Part model, mm, in its own coordinate system. A direction names the side the tool comes from. Give positions to 0.01 mm unless a question says otherwise; leave off trailing zeros. Order: outer loops, then holes, each group sorted by start corner. A loop starts at its lowest first (then second) coordinate and runs counter-clockwise, first axis right, second up. Notation, with made-up numbers: (70, -28) - (93, -28) arc R17 ccw to (93, -9) - close; hole circle Ø11 at (40, -1.75). An arc over 180 degrees is marked (long way). Use one line per item in the form item = value. Start each with the question number.
1. Pull direction Z, two halves, no side cores. Call faces 1 (the face through (4, -4.3, 11)), 2 (the face through (0.91, -1.11, -14.18)), 3 (the face through (4, 0, 34)), 4 (the face through (1.203, -0.599, 45.859)): +Z half, -Z half, draft (parallel to the pull), parting line (faces both ways), or undercut.
2. Drill centre lines: line 1 (Z direction, x = 4, y = 1.4); line 2 (Z direction, x = 7, y = -2.5); line 3 (Y direction, x = 5.25, z = -23.5). Where is each one in solid material? Low to high.
3. Tool access for faces 5 (the face through (4.195, -2.12, 14.502)), 6 (the face through (3.317, 2.696, 39.925)), 7 (the face through (4, -4.3, 41)), 8 (the face through (5, -4.3, -14)): list every direction of +Z, -Z, +X, -X, +Y, -Y with a clear straight run to the whole face (end or side of a thin tool).
4. Band-saw the part on B-B, the plane z = 4.75. List the corners of the cut face in (x, y).
5. Band-saw the part on A-A, the plane z = 13. List the corners of the cut face in (x, y), plus the area to 3 significant figures.
6. Pin check, flat tips, straight feed: P1, Ø4, axis at y = -5.5, z = 16, coming from the -X side; P2, Ø4, axis at x = 2.5, z = -21.5, coming from the -Y side. Stop position of each tip, or through.
from build123d import *

# Parameters (mm, degrees)
F0_R      = 1.5
F3_DEPTH  = 3
F0_R_2    = 3.15
F5_DEPTH  = 3
F6_DEPTH  = 4.3
F7_DEPTH  = 7.8
F8_DEPTH  = 0.8
F1_R      = 2.25
F9_DEPTH  = 88
F10_DEPTH = 0.8
F12_R     = 1
F13_DEPTH = 2.4


# Not quite as in the source:
# - an extrude ends at something that could not be found from the text; its depth is read off the source's solid


with BuildPart() as f3:
    # F0 (on Front) → F3 (new body)
    with BuildSketch(Plane.XZ):
        with BuildLine():
            Line((8.25, -28), (8.25, 0))
            Line((8.25, 0), (0, 0))
            ThreePointArc((0, 0), (0.9337479911, -14.3772966716), (3.7193040011, -28.5130394045))
            ThreePointArc((3.7193040011, -28.5130394045), (4.4329720676, -29.5852568891), (5.6523820051, -30))
            Line((5.6523820051, -30), (6.25, -30))
            ThreePointArc((6.25, -30), (7.6642135624, -29.4142135624), (8.25, -28))
        make_face()
        with Locations((4.125, -5)):
            Circle(F0_R, mode=Mode.SUBTRACT)
    extrude(amount=-F3_DEPTH)

    # F4: sweep along a path in F4_path
    with BuildLine(Plane(origin=(3.7193040011, 3, -28.5130394045), x_dir=(0, 0, 1), z_dir=(0, -1, 0))) as f4_path:
        ThreePointArc((28.5130394045, 3.7193040011), (14.1357427329, 2.78555601), (0, 0))
        ThreePointArc((0, 0), (-1.0722174846, -0.7136680665), (-1.4869605955, -1.933078004))
        Line((-1.4869605955, -1.933078004), (-1.4869605955, -2.5306959989))
        ThreePointArc((-1.4869605955, -2.5306959989), (-0.9011741579, -3.9449095613), (0.5130394045, -4.5306959989))
        Line((0.5130394045, -4.5306959989), (28.5130394045, -4.5306959989))
    # F2 (on Top) → F4 (sweep, cut)
    with BuildSketch(Plane.XY):
        with BuildLine():
            ThreePointArc((7.25, 3), (7.9571067812, 2.7071067812), (8.25, 2))
            Line((8.25, 2), (8.25, 3))
            Line((8.25, 3), (7.25, 3))
        make_face()
    sweep(path=f4_path.line, mode=Mode.SUBTRACT)

    # F0 (on Front) → F5 (join, through all)
    with BuildSketch(Plane.XZ):
        with BuildLine():
            Line((8.25, 0), (8.25, 15.324121816))
            ThreePointArc((8.25, 15.324121816), (4.1356957298, 14.5011227991), (0, 15.2088288402))
            Line((0, 15.2088288402), (0, 0))
            Line((0, 0), (8.25, 0))
        make_face()
        with BuildLine():
            Line((8.25, 15.324121816), (8.25, 23.4068600115))
            ThreePointArc((8.25, 23.4068600115), (4.2412321866, 21.0070929888), (0, 22.9669528523))
            Line((0, 22.9669528523), (0, 15.2088288402))
            ThreePointArc((0, 15.2088288402), (4.1356957298, 14.5011227991), (8.25, 15.324121816))
        make_face()
        with BuildLine():
            Line((8.25, 23.4068600115), (8.25, 26))
            Line((8.25, 26), (7.95, 26))
            ThreePointArc((7.95, 26), (3.975, 22.025), (0, 26))
            Line((0, 26), (0, 22.9669528523))
            ThreePointArc((0, 22.9669528523), (4.2412321866, 21.0070929888), (8.25, 23.4068600115))
        make_face()
        with BuildLine():
            ThreePointArc((7.95, 26), (3.975, 29.975), (0, 26))
            ThreePointArc((0, 26), (3.975, 22.025), (7.95, 26))
        make_face()
        with Locations((3.975, 26)):
            Circle(F0_R, mode=Mode.SUBTRACT)
        with Locations((3.975, 26)):
            Circle(F0_R)
        with BuildLine():
            Line((8.25, 26), (8.25, 28.5931399885))
            ThreePointArc((8.25, 28.5931399885), (4.2412321866, 30.9929070112), (0, 29.0330471477))
            Line((0, 29.0330471477), (0, 26))
            ThreePointArc((0, 26), (3.975, 29.975), (7.95, 26))
            Line((7.95, 26), (8.25, 26))
        make_face()
        with BuildLine():
            Line((8.25, 28.5931399885), (8.25, 36.675878184))
            ThreePointArc((8.25, 36.675878184), (4.1356957298, 37.4988772009), (0, 36.7911711598))
            Line((0, 36.7911711598), (0, 29.0330471477))
            ThreePointArc((0, 29.0330471477), (4.2412321866, 30.9929070112), (8.25, 28.5931399885))
        make_face()
        with BuildLine():
            Line((8.25, 47), (4, 47))
            ThreePointArc((4, 47), (1.1715728753, 45.8284271247), (0, 43))
            Line((0, 43), (0, 36.7911711598))
            ThreePointArc((0, 36.7911711598), (4.1356957298, 37.4988772009), (8.25, 36.675878184))
            Line((8.25, 36.675878184), (8.25, 47))
        make_face()
        with Locations((4, 43)):
            Circle(F0_R_2, mode=Mode.SUBTRACT)
    extrude(amount=-F5_DEPTH)

    # F0 (on Front) → F6 (join)
    with BuildSketch(Plane.XZ):
        with BuildLine():
            Line((8.25, 47), (4, 47))
            ThreePointArc((4, 47), (1.1715728753, 45.8284271247), (0, 43))
            Line((0, 43), (0, 36.7911711598))
            ThreePointArc((0, 36.7911711598), (4.1356957298, 37.4988772009), (8.25, 36.675878184))
            Line((8.25, 36.675878184), (8.25, 47))
        make_face()
        with Locations((4, 43)):
            Circle(F0_R_2, mode=Mode.SUBTRACT)
        with BuildLine():
            Line((8.25, -28), (8.25, 0))
            Line((8.25, 0), (0, 0))
            ThreePointArc((0, 0), (0.9337479911, -14.3772966716), (3.7193040011, -28.5130394045))
            ThreePointArc((3.7193040011, -28.5130394045), (4.4329720676, -29.5852568891), (5.6523820051, -30))
            Line((5.6523820051, -30), (6.25, -30))
            ThreePointArc((6.25, -30), (7.6642135624, -29.4142135624), (8.25, -28))
        make_face()
        with Locations((4.125, -5)):
            Circle(F0_R, mode=Mode.SUBTRACT)
        with Locations((3.975, 26)):
            Circle(F0_R)
        with BuildLine():
            Line((8.25, 0), (8.25, 15.324121816))
            ThreePointArc((8.25, 15.324121816), (4.1356957298, 14.5011227991), (0, 15.2088288402))
            Line((0, 15.2088288402), (0, 0))
            Line((0, 0), (8.25, 0))
        make_face()
        with Locations((4, 43)):
            Circle(F0_R_2)
        with Locations((4, 43)):
            Circle(F0_R, mode=Mode.SUBTRACT)
    extrude(amount=F6_DEPTH)

    # F0 (on Front) → F7 (join)
    with BuildSketch(Plane.XZ):
        with BuildLine():
            ThreePointArc((7.95, 26), (3.975, 29.975), (0, 26))
            ThreePointArc((0, 26), (3.975, 22.025), (7.95, 26))
        make_face()
        with Locations((3.975, 26)):
            Circle(F0_R, mode=Mode.SUBTRACT)
    extrude(amount=F7_DEPTH)

    # F0 (on Front) → F8 (join)
    with BuildSketch(Plane.XZ):
        with BuildLine():
            Line((8.25, 26), (8.25, 28.5931399885))
            ThreePointArc((8.25, 28.5931399885), (4.2412321866, 30.9929070112), (0, 29.0330471477))
            Line((0, 29.0330471477), (0, 26))
            ThreePointArc((0, 26), (3.975, 29.975), (7.95, 26))
            Line((7.95, 26), (8.25, 26))
        make_face()
    extrude(amount=F8_DEPTH)

    # F1 (on Right) → F9 (cut, through all)
    with BuildSketch(Plane.YZ):
        with Locations((-4.3, 4.75)):
            Circle(F1_R)
    extrude(amount=F9_DEPTH, mode=Mode.SUBTRACT)

    # F0 (on Front) → F10 (join)
    with BuildSketch(Plane.XZ):
        with BuildLine():
            Line((8.25, 23.4068600115), (8.25, 26))
            Line((8.25, 26), (7.95, 26))
            ThreePointArc((7.95, 26), (3.975, 22.025), (0, 26))
            Line((0, 26), (0, 22.9669528523))
            ThreePointArc((0, 22.9669528523), (4.2412321866, 21.0070929888), (8.25, 23.4068600115))
        make_face()
    extrude(amount=F10_DEPTH)

    # F2 (on Top) → F11 (revolve, cut)
    with BuildSketch(Plane.XY):
        with BuildLine():
            ThreePointArc((7.25, 3), (7.9571067812, 2.7071067812), (8.25, 2))
            Line((8.25, 2), (8.25, 3))
            Line((8.25, 3), (7.25, 3))
        make_face()
    revolve(axis=Axis((7.75, 3, 0), (-1, 0, 0)), mode=Mode.SUBTRACT)

    # F12
    f12_edges = [f3.edges().sort_by_distance(p)[0] for p in [
        (8.25, -0.65, 47),
    ]]
    fillet(f12_edges, radius=F12_R)

    # F0 (on Front) → F13 (join)
    with BuildSketch(Plane.XZ):
        with Locations((4, 43)):
            Circle(F0_R_2)
        with Locations((4, 43)):
            Circle(F0_R, mode=Mode.SUBTRACT)
    extrude(amount=-F13_DEPTH)


solid = f3.part
From the geometry:
q1.face_1 = draft
q1.face_2 = -Z half
q1.face_3 = undercut
q1.face_4 = +Z half
q2.line_1 = -29.13 to -6.49, -3.51 to 41.5, 44.5 to 47
q2.line_2 = -29.85 to 3.4, 6.1 to 14.9, 23.42 to 28.58, 37.1 to 47
q2.line_3 = -4.3 to 3
q3.face_5 = -Y
q3.face_6 = +Y
q3.face_7 = +Z, +X, -X, -Y
q3.face_8 = -Z, +X, -X, -Y
q4.outline = (0, -2.05) - (8.25, -2.05) - (8.25, 3) - (0, 3) - close
q5.outline = (0, -4.3) - (8.25, -4.3) - (8.25, 3) - (0, 3) - close
q5.area = 60.2 mm²
q6.P1 = 0
q6.P2 = -4.3
